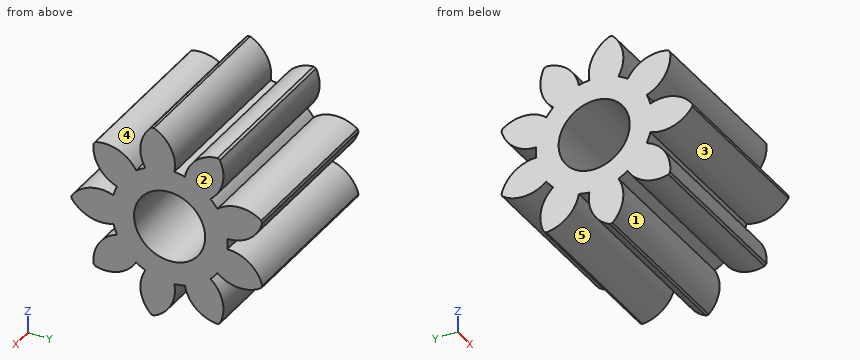
from build123d import *

# Parameters (mm, degrees)
BASPROSKE_W              = 12
BASPROSKE_H              = 6.9
TOOTHCUT_DEPTH           = 16.466738506
PATTERN_CIRCULAR_1_COUNT = 9
SKETCH_1_R               = 2.5
CUT_EXTRUDE_1_DEPTH      = 16.427377744
SCALE_1_SCALE            = 1.03


with BuildPart() as part:
    # BasProSke → Base-Revolve (revolve)
    with BuildSketch(Plane(origin=(0, 0, 0), x_dir=(1, 0, 0), z_dir=(0, 1, 0)), mode=Mode.PRIVATE) as base_revolve_sk:
        with Locations((6, 3.45)):
            Rectangle(BASPROSKE_W, BASPROSKE_H)
    revolve(base_revolve_sk.sketch.rotate(Axis((-10, 0, 0), (1, 0, 0)), 180), axis=Axis((-10, 0, 0), (1, 0, 0)))

    # TooCutSke → ToothCut (cut, through all)
    with BuildSketch(Plane(origin=(0, 0, 0), x_dir=(0, 0, -1), z_dir=(1, 0, 0))):
        with BuildLine():
            ThreePointArc((0.374882812, 4.069268377), (0, 4.0865), (-0.374882812, 4.069268377))
            ThreePointArc((-0.374882812, 4.069268377), (-0.912200879, 5.63954288), (-2.314462256, 6.527312978))
            ThreePointArc((-2.314462256, 6.527312978), (0, 6.9255), (2.314462256, 6.527312978))
            ThreePointArc((2.314462256, 6.527312978), (0.912200879, 5.63954288), (0.374882812, 4.069268377))
        make_face()
    toothcut = extrude(amount=TOOTHCUT_DEPTH, mode=Mode.SUBTRACT)

    # Круговой массив1: ToothCut ×9 about axis
    pattern_circular_1_axis = Axis((0, 0, 0), (1, 0, 0))
    for i in range(1, PATTERN_CIRCULAR_1_COUNT):
        add(toothcut.rotate(pattern_circular_1_axis, i * 360 / PATTERN_CIRCULAR_1_COUNT), mode=Mode.SUBTRACT)

    # Эскиз1 → Вырез-Вытянуть1 (cut, through all)
    with BuildSketch(Plane(origin=(12, 0, 0), x_dir=(0, 0, -1), z_dir=(1, 0, 0))):
        Circle(SKETCH_1_R)
    extrude(amount=-CUT_EXTRUDE_1_DEPTH, mode=Mode.SUBTRACT)


with BuildPart() as part_1:
    # Масштаб1: scaled about (6, 0, 0)
    add(part.part.scale(SCALE_1_SCALE).moved(Location((-0.18, 0, 0))))


solid = part_1.part
Check sheet for the modelled part. Datum: model origin and axes. Units: mm. Face numbers are marked on the shaded views. A direction names the side the tool comes from. Give positions to 0.01 mm unless a question says otherwise; leave off trailing zeros. Loops run counter-clockwise (first coordinate to the right, second up) from the corner with the lowest first, then second, coordinate; pieces in that order, holes last. Notation, with made-up numbers: M 74.5,-23.75 L 131.5,-23.75 A25 ccw 131.5,2.25 Z; hole C 53.25,4.5 d4. An arc over 180 degrees is marked long. Use a Markdown table: item, result. Add a question column.
Q1. Scan lines: line 1 along Y through (x, z) = (4.5, 0) (3 decimals); line 2 along Y through (x, z) = (1, 6); line 3 along Z through (x, y) = (0.5, 5). Record each from-to range of solid material in increasing order. Write a range as [from, to].
Q2. Mould release check, pull along Z, two halves, no side actions. Record for the marked faces 1 and 2: pulls with the +Z half, pulls with the -Z half, needs draft (parallel to the pull), parting line crosses it, or undercut.
Q3. Go/stop test with flat-tipped pins: pin 1 (3 mm diameter, centred on x = 5, y = 5, fed in from +Z); pin 2 (4.5 mm diameter, centred on y = 0, z = 0, fed in from -X); pin 3 (4 mm diameter, centred on x = 4, y = 4, fed in from -Z). Record where each tip stops, or that it passes through.
Q4. Sectioned sample at C-C, the plane z = -0.75. Record the cut outline in (x, y), then the cut area to 3 significant figures.
Q5. Tool access check on the marked faces 3, 4 and 5. Record the directions out of +Z, -Z, +X, -X, +Y, -Y that give a thin tool (end or side, any length) a straight path to the whole face; none if there is none.
Q6. Sectioned sample at B-B, the plane y = 0. Record the cut outline in (x, z) (3 decimals).
Q7. Sectioned sample at A-A, the plane y = -5. Record the cut outline in (x, z), then the cut area to 3 significant figures.
Verdict:
| question | item | result |
|---|---|---|
| 1 | line 1 | [-7.107, -2.575], [2.575, 4.209] |
| 1 | line 2 | [-1.97, 0.02], [2.63, 3.69] |
| 1 | line 3 | [-3.01, -0.51], [0.51, 3.01] |
| 2 | face 1 | undercut |
| 2 | face 2 | needs draft |
| 3 | pin 1 | z = 6.19 |
| 3 | pin 2 | through |
| 3 | pin 3 | z = -6.2 |
| 4 | outline | M -0.18,-6.47 L 12.18,-6.47 L 12.18,-2.46 L -0.18,-2.46 Z; M -0.18,2.46 L 12.18,2.46 L 12.18,5.53 L -0.18,5.53 Z |
| 4 | area | 87.5 mm^2 |
| 5 | face 3 | +X, -X |
| 5 | face 4 | +Z, +X, -X |
| 5 | face 5 | -Z, +X, -X |
| 6 | outline | M -0.18,-6.027 L 12.18,-6.027 L 12.18,-2.575 L -0.18,-2.575 Z; M -0.18,2.575 L 12.18,2.575 L 12.18,6.027 L -0.18,6.027 Z |
| 7 | outline | M -0.18,-4.72 L 12.18,-4.72 L 12.18,-2.67 L -0.18,-2.67 Z; M -0.18,-1.23 L 12.18,-1.23 L 12.18,1.23 L -0.18,1.23 Z; M -0.18,2.67 L 12.18,2.67 L 12.18,4.72 L -0.18,4.72 Z |
| 7 | area | 81.2 mm^2 |
